from build123d import *

# Parameters (mm, degrees)
BOX003_W               = 95
BOX003_H               = 48
BOX003_DEPTH           = 2
BOX004_W               = 95
BOX004_H               = 48
BOX004_DEPTH           = 2
BOX004_PLACEMENT_ANGLE = 90
BOX002_W               = 50
BOX002_H               = 13
BOX002_DEPTH           = 39
BOX001_W               = 56
BOX001_H               = 46
BOX001_DEPTH           = 59
BOX_W                  = 58
BOX_H                  = 48
BOX_DEPTH              = 50


with BuildPart() as cube003:
    # Box003 → Box003 (new body)
    with BuildSketch(Plane(origin=(-18, 0, 0), x_dir=(1, 0, 0), z_dir=(0, 0, 1))):
        with Locations((47.5, 24)):
            Rectangle(BOX003_W, BOX003_H)
    extrude(amount=BOX003_DEPTH)


with BuildPart() as cube004:
    # Box004 → Box004 (new body)
    with BuildSketch(Plane.XY):
        with Locations((47.5, 24)):
            Rectangle(BOX004_W, BOX004_H)
    extrude(amount=BOX004_DEPTH)


with BuildPart() as cube004_1:
    # Box004 placement: moved
    add(cube004.part.moved(Location((54, -22, 0))).rotate(Axis((54, -22, 0), (0, 0, 1)), BOX004_PLACEMENT_ANGLE))


with BuildPart() as cube002:
    # Box002 → Box002 (new body)
    with BuildSketch(Plane(origin=(4, -2, 7), x_dir=(1, 0, 0), z_dir=(0, 0, 1))):
        with Locations((25, 6.5)):
            Rectangle(BOX002_W, BOX002_H)
    extrude(amount=BOX002_DEPTH)


with BuildPart() as cube001:
    # Box001 → Box001 (new body)
    with BuildSketch(Plane(origin=(1, 1, 2), x_dir=(1, 0, 0), z_dir=(0, 0, 1))):
        with Locations((28, 23)):
            Rectangle(BOX001_W, BOX001_H)
    extrude(amount=BOX001_DEPTH)


with BuildPart() as fusion:
    # Box → Box (new body)
    with BuildSketch(Plane.XY):
        with Locations((29, 24)):
            Rectangle(BOX_W, BOX_H)
    extrude(amount=BOX_DEPTH)

    # Cut: cut Cube001
    add(cube001.part, mode=Mode.SUBTRACT)

    # Cut001: cut Cube002
    add(cube002.part, mode=Mode.SUBTRACT)

    # Fusion: union Cube003, Cube004
    add(cube003.part)
    add(cube004_1.part)


solid = fusion.part
Here's how the part is built. I have some questions about the finished solid (model axes, mm). A direction names the side the tool comes from. Coordinates: 2 decimals unless noted, no trailing zeros. Order: outer loops, then holes, each group sorted by start corner. A loop starts at its lowest first (then second) coordinate and runs counter-clockwise, first axis right, second up.
Item 1: If we section it at B-B on z = 4: List the corners of the cut face in (x, y) for me.
Result sheet:
outline: (0, 0) - (58, 0) - (58, 48) - (0, 48) - close; hole (1, 1) - (57, 1) - (57, 47) - (1, 47) - close
Item 2: I need wall thicknesses on line 1 (X direction, y = 36.5, z = 40); line 2 (Y direction, x = 45, z = 47); line 3 (Y direction, x = 8.5, z = 41). Which ranges of each line are inside material? Lowest first, please.
Result sheet:
line 1: x = 0 to 1, 57 to 58
line 2: y = 0 to 1, 47 to 48
line 3: y = 47 to 48
Item 3: If we mould it in two halves opening along X, with no side actions, what happens to faces 1 (the face through (0, 24, 26)), 2 (the face through (29, 25, 0)), 3 (the face through (25, 1, 6)), 4 (the face through (1, 24, 26))? For each: +X half, -X half, draft (parallel to the pull), parting line (faces both ways), or undercut.
Result sheet:
face 1: -X half
face 2: draft
face 3: undercut
face 4: undercut
Item 4: For faces 5 (the face through (30, -11, 2)), 6 (the face through (-9, 24, 2)), 7 (the face through (29, 24, 2)), 8 (the face through (30, 60, 2)), 9 (the face through (67, 24, 2)), which set-ups out of +Z, -Z, +X, -X, +Y, -Y let a thin tool reach every point of the face, with its end or its side?
Result sheet:
face 5: +Z, +X, -X, -Y
face 6: +Z, -X, +Y, -Y
face 7: +Z
face 8: +Z, +X, -X, +Y
face 9: +Z, +X, +Y, -Y
Item 5: If we section it at C-C on y = 11: List the corners of the cut face in (x, z) for me, plus the area to 3 significant figures.
Result sheet:
outline: (-18, 0) - (77, 0) - (77, 2) - (58, 2) - (58, 50) - (57, 50) - (57, 2) - (1, 2) - (1, 50) - (0, 50) - (0, 2) - (-18, 2) - close
area: 286 mm2
Item 6: If we section it at D-D on z = 33: List the corners of the cut face in (x, y) for me.
Result sheet:
outline: (0, 0) - (4, 0) - (4, 1) - (1, 1) - (1, 47) - (57, 47) - (57, 1) - (54, 1) - (54, 0) - (58, 0) - (58, 48) - (0, 48) - close
Item 7: For P1, Ø1.1, axis at y = 0.5, z = 24.5, coming from the +X side; P2, Ø2, axis at x = 19, z = 16, coming from the -Y side; P3, Ø1.5, axis at x = 7.5, z = 20, coming from the +Y side, each with a flat end and sliding along its axis, tell me the tip position at first contact or that it passes through.
Result sheet:
P1: stops at x = 58
P2: stops at y = 47
P3: stops at y = 48
Item 8: If we section it at A-A on x = 43: List the corners of the cut face in (y, z) for me.
Result sheet:
outline: (-22, 0) - (73, 0) - (73, 2) - (48, 2) - (48, 50) - (47, 50) - (47, 2) - (1, 2) - (1, 7) - (0, 7) - (0, 2) - (-22, 2) - close; (0, 46) - (1, 46) - (1, 50) - (0, 50) - close
